from build123d import *

# Parameters (mm, degrees)
SKETCH_1_W          = 8
SKETCH_1_H          = 10
SKETCH_2_R          = 5
EXTRUDE_1_DEPTH     = 88
CUT_EXTRUDE_1_DEPTH = 7
CHAMFER_1_SIZE2     = 1.000000001
CHAMFER_1_SIZE      = 0.999999999


with BuildPart() as part:
    # 草图1 → 旋转1 (revolve)
    with BuildSketch(Plane(origin=(0, 0, 0), x_dir=(1, 0, 0), z_dir=(0, 1, 0))):
        with Locations((4, -5)):
            Rectangle(SKETCH_1_W, SKETCH_1_H)
    revolve(axis=Axis((0, 0, 0), (0, 0, 1)))

    # 草图2 → 凸台-拉伸1 (add)
    with BuildSketch(Plane.XY.offset(10)):
        Circle(SKETCH_2_R)
    extrude(amount=EXTRUDE_1_DEPTH)

    # 草图3 → 切除-拉伸1 (cut)
    with BuildSketch(Plane(origin=(0, 0, 0), x_dir=(-1, 0, 0), z_dir=(0, 0, -1))):
        Polygon((-2.309401077, 4), (-4.618802154, 0), (-2.309401077, -4), (2.309401077, -4), (4.618802154, 0), (2.309401077, 4), align=None)
    extrude(amount=-CUT_EXTRUDE_1_DEPTH, mode=Mode.SUBTRACT)

    # 倒角1
    chamfer_1_edges = [part.edges().sort_by_distance(p)[0] for p in [
        (-5, 0, 98),
        (-8, 0, 0),
    ]]
    chamfer(chamfer_1_edges, length=CHAMFER_1_SIZE, length2=CHAMFER_1_SIZE2)


solid = part.part
Source: CAD feature listing. Evaluate the final solid. Frame: model axes, mm. A direction names the side the tool comes from. Coordinates: 2 decimals unless noted, no trailing zeros. Loops run counter-clockwise (first coordinate to the right, second up) from the corner with the lowest first, then second, coordinate; pieces in that order, holes last. Notation, with made-up numbers: (24.5, 58) - (78.5, 58) arc R19 ccw to (78.5, 78) - close; hole circle Ø11 at (46.5, 85.5). An arc over 180 degrees is marked (long way). One line per item, written item: value. Start each with the question number.
1. Section A-A (x = 0). Return the cut outline in (y, z).
2. Section B-B (z = 71). Return the cut outline in (x, y), and give its area (3 significant figures).
3. Set-up query: faces 1 (the flat face through (-5, 0, 0)), 2 (the flat face through (0.1, -5.2, 10)), 3 (the flat face through (0, 0, 7)). Return all of +Z, -Z, +X, -X, +Y, -Y with unobstructed straight access to the full face (end or side cutting, diameter ignored); none if empty.
4. Contact query for flat-ended pins moving along their axis: P1, Ø5, axis at x = -3.5, z = 27.5, coming from the +Y side; P2, Ø1, axis at x = -3, z = 22.5, coming from the -Y side; P3, Ø6.5, axis at x = 0.5, y = -1.5, coming from the -Z side; P4, Ø1, axis at y = -4.5, z = 65.5, coming from the -X side. Output: stop coordinate, or through.
5. Mould query, pull axis Y, two halves, no side actions, for faces 4 (the flat face through (0, 0, 98)), 5 (the cylindrical face through (-1.73, -7.81, 5.44)), 6 (the flat face through (0, 4, 3)). Classes: pulls with the +Y half, pulls with the -Y half, needs draft (parallel to the pull), parting line crosses it, or undercut.
6. Ray query, L1, parallel to Z at x = 1.5, y = 1.75; L2, parallel to Z at x = 1.25, y = 6.75; L3, parallel to Y at x = 0.25, z = 24. Return the intervals inside material, ascending.
Verdict:
1. outline: (-8, 1) - (-7, 0) - (-4, 0) - (-4, 7) - (4, 7) - (4, 0) - (7, 0) - (8, 1) - (8, 10) - (5, 10) - (5, 97) - (4, 98) - (-4, 98) - (-5, 97) - (-5, 10) - (-8, 10) - close
2. outline: circle Ø10 at (0, 0)
2. area: 78.5 mm2
3. face 1: -Z, +X, -X, +Y, -Y
3. face 2: +Z
3. face 3: -Z
4. P1: stops at y = 4.9
4. P2: stops at y = -4.33
4. P3: stops at z = 0
4. P4: stops at x = -3
5. face 4: needs draft
5. face 5: parting line crosses it
5. face 6: undercut
6. L1: z = 7 to 98
6. L2: z = 0 to 10
6. L3: y = -4.99 to 4.99
